```python
from build123d import *

# Parameters (mm, degrees)
BOSS_EXTRU_1_DEPTH         = 6.35
ESQUISSE4_W                = 6.35
ESQUISSE4_H                = 10.16
ESQUISSE4_W_2              = 6.472054313
ENL_V_MAT_EXTRU_1_DEPTH    = 237.318984637
R_P_TITION_LIN_AIRE3_COUNT = 3
R_P_TITION_LIN_AIRE3_PITCH = 20.32
ESQUISSE6_W                = 25.4
ESQUISSE6_H                = 6.35
BOSS_EXTRU_3_DEPTH         = 6.35
R_P_TITION_LIN_AIRE4_COUNT = 7
R_P_TITION_LIN_AIRE4_PITCH = 50.8
ESQUISSE7_W                = 6.35
ESQUISSE7_H                = 10.16
ENL_V_MAT_EXTRU_2_DEPTH    = 6.35
ESQUISSE8_W                = 12.7
ESQUISSE8_H                = 6.35
ENL_V_MAT_EXTRU_3_DEPTH    = 6.35
R_P_TITION_LIN_AIRE6_COUNT = 5
R_P_TITION_LIN_AIRE6_PITCH = 25.4
ESQUISSE9_W                = 6.35
ESQUISSE9_H                = 25.4
ENL_V_MAT_EXTRU_4_DEPTH    = 6.35
R_P_TITION_LIN_AIRE7_COUNT = 3
R_P_TITION_LIN_AIRE7_PITCH = 50.8
ESQUISSE10_W               = 6.35
ESQUISSE10_H               = 12.7
ENL_V_MAT_EXTRU_5_DEPTH    = 6.35
SKETCH1_W                  = 120.65
SKETCH1_H                  = 57.15
CUT_EXTRUDE1_DEPTH         = 237.318984637
ENL_V_MAT_EXTRU_6_REACH    = 238.319
ESQUISSE11_R               = 6.35


with BuildPart() as part:
    # Esquisse1 → Boss.-Extru.1 (new body)
    with BuildSketch(Plane(origin=(0, 0, 0), x_dir=(0, 0, -1), z_dir=(1, 0, 0))):
        Polygon((-57.15, 38.1), (-57.15, 88.9), (63.5, 88.9), (63.5, 139.7), (190.5, 139.7), (190.5, -12.7), (-177.8, -12.7), (-177.8, 38.1), align=None)
    extrude(amount=BOSS_EXTRU_1_DEPTH)

    # Esquisse4 → Enlèv. mat.-Extru.1 (cut, through all)
    with BuildSketch(Plane(origin=(6.35, 0, 0), x_dir=(0, 0, -1), z_dir=(1, 0, 0))):
        with Locations((-174.625, -7.62)):
            Rectangle(ESQUISSE4_W, ESQUISSE4_H)
        with Locations((-53.975, 43.18)):
            Rectangle(ESQUISSE4_W, ESQUISSE4_H)
        with Locations((66.736027157, 93.98)):
            Rectangle(ESQUISSE4_W_2, ESQUISSE4_H)
    enl_v_mat_extru_1 = extrude(amount=-ENL_V_MAT_EXTRU_1_DEPTH, mode=Mode.SUBTRACT)

    # Répétition linéaire3: Enlèv. mat.-Extru.1 ×3
    with Locations(*[(0, i * R_P_TITION_LIN_AIRE3_PITCH, 0) for i in range(1, R_P_TITION_LIN_AIRE3_COUNT)]):
        add(enl_v_mat_extru_1, mode=Mode.SUBTRACT)

    # Esquisse6 → Boss.-Extru.3 (add)
    with BuildSketch(Plane(origin=(6.35, 0, 0), x_dir=(0, 0, -1), z_dir=(1, 0, 0))):
        with Locations((-142.875, -15.875)):
            Rectangle(ESQUISSE6_W, ESQUISSE6_H)
    boss_extru_3 = extrude(amount=-BOSS_EXTRU_3_DEPTH)

    # Répétition linéaire4: Boss.-Extru.3 ×7
    with Locations(*[(0, 0, -i * R_P_TITION_LIN_AIRE4_PITCH) for i in range(1, R_P_TITION_LIN_AIRE4_COUNT)]):
        add(boss_extru_3)

    # Esquisse7 → Enlèv. mat.-Extru.2 (cut)
    with BuildSketch(Plane(origin=(6.35, 0, 0), x_dir=(0, 0, -1), z_dir=(1, 0, 0))):
        with Locations((-53.975, 22.86)):
            Rectangle(ESQUISSE7_W, ESQUISSE7_H)
        with Locations((66.797054313, 73.66)):
            Rectangle(ESQUISSE7_W, ESQUISSE7_H)
        with Locations((-53.975, 2.54)):
            Rectangle(ESQUISSE7_W, ESQUISSE7_H)
        with Locations((66.797054313, 53.34)):
            Rectangle(ESQUISSE7_W, ESQUISSE7_H)
    extrude(amount=-ENL_V_MAT_EXTRU_2_DEPTH, mode=Mode.SUBTRACT)

    # Esquisse8 → Enlèv. mat.-Extru.3 (cut)
    with BuildSketch(Plane(origin=(6.35, 0, 0), x_dir=(0, 0, -1), z_dir=(1, 0, 0))):
        with Locations((-38.1, 34.925)):
            Rectangle(ESQUISSE8_W, ESQUISSE8_H)
        with Locations((82.672054313, 85.725)):
            Rectangle(ESQUISSE8_W, ESQUISSE8_H)
    enl_v_mat_extru_3 = extrude(amount=-ENL_V_MAT_EXTRU_3_DEPTH, mode=Mode.SUBTRACT)

    # Répétition linéaire6: Enlèv. mat.-Extru.3 ×5
    with Locations(*[(0, 0, -i * R_P_TITION_LIN_AIRE6_PITCH) for i in range(1, R_P_TITION_LIN_AIRE6_COUNT)]):
        add(enl_v_mat_extru_3, mode=Mode.SUBTRACT)

    # Esquisse9 → Enlèv. mat.-Extru.4 (cut)
    with BuildSketch(Plane(origin=(6.35, 0, 0), x_dir=(0, 0, -1), z_dir=(1, 0, 0))):
        with Locations((187.325, 88.9)):
            Rectangle(ESQUISSE9_W, ESQUISSE9_H)
    enl_v_mat_extru_4 = extrude(amount=-ENL_V_MAT_EXTRU_4_DEPTH, mode=Mode.SUBTRACT)

    # Répétition linéaire7: Enlèv. mat.-Extru.4 ×3
    with Locations(*[(0, -i * R_P_TITION_LIN_AIRE7_PITCH, 0) for i in range(1, R_P_TITION_LIN_AIRE7_COUNT)]):
        add(enl_v_mat_extru_4, mode=Mode.SUBTRACT)

    # Esquisse10 → Enlèv. mat.-Extru.5 (cut)
    with BuildSketch(Plane(origin=(6.35, 0, 0), x_dir=(0, 0, -1), z_dir=(1, 0, 0))):
        with Locations((187.325, 133.35)):
            Rectangle(ESQUISSE10_W, ESQUISSE10_H)
    extrude(amount=-ENL_V_MAT_EXTRU_5_DEPTH, mode=Mode.SUBTRACT)

    # Sketch1 → Cut-Extrude1 (cut, through all)
    with BuildSketch(Plane(origin=(6.35, 0, 0), x_dir=(0, 0, -1), z_dir=(1, 0, 0))):
        with Locations((-117.475, 9.525)):
            Rectangle(SKETCH1_W, SKETCH1_H)
    extrude(amount=-CUT_EXTRUDE1_DEPTH, mode=Mode.SUBTRACT)

    # Esquisse11 → Enlèv. mat.-Extru.6 (cut, up to next)
    with BuildSketch(Plane.ZY, mode=Mode.PRIVATE) as enl_v_mat_extru_6_sk1:
        with Locations((-66.675, 6.35)):
            Circle(ESQUISSE11_R)
    enl_v_mat_extru_6_tool1 = extrude(enl_v_mat_extru_6_sk1.sketch, amount=-ENL_V_MAT_EXTRU_6_REACH, mode=Mode.PRIVATE) & part.part
    add(enl_v_mat_extru_6_tool1.solids().sort_by_distance((0, 6.35, -66.675))[0], mode=Mode.SUBTRACT)


solid = part.part
```
CAD build for the part. Positions are in the model's coordinates, mm. A direction names the side the tool comes from. Round coordinates to 2 decimals unless told otherwise and drop trailing zeros. Order: outer loops, then holes, each group sorted by start corner. A loop starts at its lowest first (then second) coordinate and runs counter-clockwise, first axis right, second up.
Item 1: Pin check, flat tips, straight feed: pin 1 (3 mm diameter, centred on x = 2, z = -135.5, fed in from -Y); pin 2 (2 mm diameter, centred on x = 5, z = -32.5, fed in from +Y); pin 3 (1.9 mm diameter, centred on x = 2, y = -5, fed in from -Z). Stop position of each tip, or through.
Item 2: Saw through at C-C on z = 23. Write the cut outline in (x, y).
Item 3: Saw through at A-A on y = 55. Write the cut outline in (x, z), then the cut area to 3 significant figures.
Item 4: Saw through at B-B on x = 1. State how many separate pieces and enclosed holes the cut face has, then the cut area to 3 significant figures.
Item 5: Tool access for faces 1 (the face through (3, 27.94, 54)), 2 (the face through (3, 88.9, -108)), 3 (the face through (3, -16, -47.625)): list every direction of +Z, -Z, +X, -X, +Y, -Y with a clear straight run to the whole face (end or side of a thin tool).
Item 6: Mould opens along Y. For faces 4 (the face through (3, -19.05, -162)), 5 (the face through (3, -16, -98.425)), 6 (the face through (3, 58.42, 54)) say: pulls with the +Y half, pulls with the -Y half, needs draft (parallel to the pull), parting line crosses it, or undercut.
Item 7: Probe line 1 along Z through (x, y) = (4.75, 88.5); line 2 along Y through (x, z) = (2, -132.5); line 3 along Y through (x, z) = (5, -61). List the from-to ranges inside material, lowest first.
Reported:
1. pin 1: stops at y = -12.7
1. pin 2: stops at y = 88.9
1. pin 3: stops at z = -184.15
2. outline: (0, -12.7) - (6.35, -12.7) - (6.35, 88.9) - (0, 88.9) - close
3. outline: (0, -190.5) - (6.35, -190.5) - (6.35, -69.97) - (0, -69.97) - close; (0, -63.62) - (6.35, -63.62) - (6.35, 57.15) - (0, 57.15) - close
3. area: 1,530 mm2
4. separate pieces: 1
4. enclosed holes: 12
4. area: 30,400 mm2
5. face 1: +Z, +X, -X
5. face 2: +X, -X
5. face 3: +X, -X, -Y
6. face 4: pulls with the -Y half
6. face 5: needs draft
6. face 6: undercut
7. line 1: z = -177.92 to -165.22, -152.52 to -139.82, -127.12 to -114.42, -101.72 to -89.02, -76.32 to 50.8
7. line 2: y = -12.7 to 82.55, 88.9 to 139.7
7. line 3: y = -19.05 to 3.5, 9.2 to 31.75, 38.1 to 88.9
